Source: three-view drawing plus pictorial views. Frame: mm from the lowest corner of the part. A direction names the side the tool comes from. Round coordinates to 2 decimals unless told otherwise and drop trailing zeros. Loops run counter-clockwise (first coordinate to the right, second up) from the corner with the lowest first, then second, coordinate; pieces in that order, holes last. Notation, with made-up numbers: (-17, 47.25) -> (-13, 47.25) arc R29 ccw to (-13, 69.25) -> close; hole circle Ø3 at (-36.5, 78.5). An arc over 180 degrees is marked (long way). Answer in a Markdown table with one row per item. Add a question column.
Q1. Reachability of the marked faces 1 and 2 from +Z, -Z, +X, -X, +Y, -Y: full face, straight path, thin tool, end or side. Return the list, or none.
Q2. Ray query, L1, parallel to Y at x = 50, z = 8.5; L2, parallel to Y at x = 49.5, z = 7.75 (1 decimal); L3, parallel to X at y = 68, z = 2. Return the intervals inside material, ascending. Write a range as from..to.
Q3. Section D-D, the plane z = 4.5. Output: boundary loops of the cut face in (x, y).
Q4. Pin query (flat end, axial travel): pin 1 (0.8 mm diameter, centred on x = 61.5, z = 1, fed in from +Y); pin 2 (1.6 mm diameter, centred on x = 50, y = 25, fed in from +Z); pin 3 (0.8 mm diameter, centred on x = 8, z = 2, fed in from -Y); pin 4 (0.8 mm diameter, centred on x = 50, y = 50, fed in from +Z). Return the tip coordinate at first contact, or that it passes through.
Q5. Section A-A, the plane y = 37.45. Output: boundary loops of the cut face in (x, z).
Q6. Section B-B, the plane z = 10.5. Output: boundary loops of the cut face in (x, y).
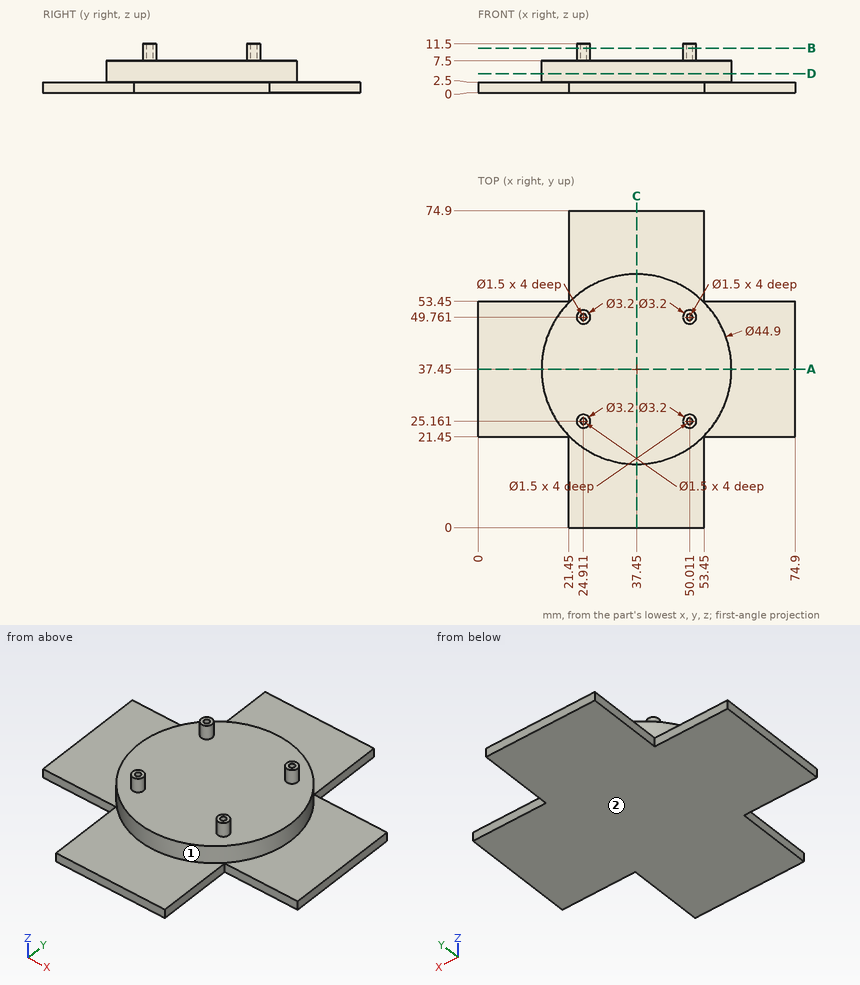
Answer block:
| question | item | result |
|---|---|---|
| 1 | face 1 | +Z |
| 1 | face 2 | -Z, +X, -X, +Y, -Y |
| 2 | L1 | 23.56..24.41, 25.91..26.76, 48.16..49.01, 50.51..51.36 |
| 2 | L2 | 23.6..24.6, 25.7..26.7, 48.2..49.2, 50.3..51.3 |
| 2 | L3 | 21.45..53.45 |
| 3 | outline | circle Ø44.9 at (37.45, 37.45) |
| 4 | pin 1 | y = 53.45 |
| 4 | pin 2 | z = 11.5 |
| 4 | pin 3 | y = 21.45 |
| 4 | pin 4 | z = 7.5 |
| 5 | outline | (0, 0) -> (74.9, 0) -> (74.9, 2.5) -> (59.9, 2.5) -> (59.9, 7.5) -> (15, 7.5) -> (15, 2.5) -> (0, 2.5) -> close |
| 6 | outline | circle Ø3.2 at (24.91, 25.16); circle Ø3.2 at (24.91, 49.76); circle Ø3.2 at (50.01, 25.16); circle Ø3.2 at (50.01, 49.76); hole circle Ø1.5 at (24.91, 25.16); hole circle Ø1.5 at (24.91, 49.76); hole circle Ø1.5 at (50.01, 25.16); hole circle Ø1.5 at (50.01, 49.76) |
